from build123d import *

# Parameters (mm, degrees)
SKETCH_1_W          = 18
SKETCH_1_H          = 18
EXTRUDE_1_DEPTH     = 25
SKETCH_2_R          = 6.55
CUT_EXTRUDE_1_DEPTH = 4.5
CUT_EXTRUDE_2_DEPTH = 11.7
CUT_EXTRUDE_3_DEPTH = 16
SKETCH_6_W          = 18
SKETCH_6_H          = 18
SKETCH_6_W_2        = 17
SKETCH_6_H_2        = 17
CUT_EXTRUDE_5_DEPTH = 26


with BuildPart() as part:
    # 草图1 → 凸台-拉伸1 (new body)
    with BuildSketch(Plane(origin=(0, 0, 0), x_dir=(0, 0, -1), z_dir=(1, 0, 0))):
        with Locations((9, 9)):
            Rectangle(SKETCH_1_W, SKETCH_1_H)
    extrude(amount=EXTRUDE_1_DEPTH)

    # 草图2 → 切除-拉伸1 (cut)
    with BuildSketch(Plane.XY):
        with Locations((10, 9)):
            Circle(SKETCH_2_R)
    extrude(amount=-CUT_EXTRUDE_1_DEPTH, mode=Mode.SUBTRACT)

    # 草图3 → 切除-拉伸2 (cut)
    with BuildSketch(Plane.XY.offset(-4.5)):
        Polygon((10, 13.618802154), (6, 11.309401077), (6, 6.690598923), (10, 4.381197846), (14, 6.690598923), (14, 11.309401077), align=None)
    extrude(amount=-CUT_EXTRUDE_2_DEPTH, mode=Mode.SUBTRACT)

    # 草图4 → 切除-拉伸3 (cut)
    with BuildSketch(Plane.XY):
        Polygon((19, 17.886751346), (16.5, 16.443375673), (16.5, 13.556624327), (19, 12.113248654), (21.5, 13.556624327), (21.5, 16.443375673), align=None)
    extrude(amount=-CUT_EXTRUDE_3_DEPTH, mode=Mode.SUBTRACT)

    # 草图6 → 切除-拉伸5 (cut, through all)
    with BuildSketch(Plane.ZY):
        with Locations((-9, 9)):
            Rectangle(SKETCH_6_W, SKETCH_6_H)
        with Locations((-9, 9)):
            Rectangle(SKETCH_6_W_2, SKETCH_6_H_2, mode=Mode.SUBTRACT)
    extrude(amount=-CUT_EXTRUDE_5_DEPTH, mode=Mode.SUBTRACT)


solid = part.part
Read the model definition and answer for the solid it produces. Units are mm, in the model's axes. A direction names the side the tool comes from. Round coordinates to 2 decimals unless told otherwise and drop trailing zeros. Write each loop counter-clockwise with the first axis right and the second up, starting at its lowest first coordinate (ties: lowest second). Pieces come first, ordered by that corner, then holes. Notation, with made-up numbers: (0, -17) - (10, -17) arc R23 ccw to (10, -7) - close; hole circle Ø7 at (23, 21.25). An arc over 180 degrees is marked (long way). Use a Markdown table: item, result.
(1) Straight lines are drawn through the part: line 1 along X through (y, z) = (11, -7.5); line 2 along X through (y, z) = (12.75, -13.5); line 3 along Y through (x, z) = (10, -3.05). For each, find the intervals that lie inside material, in ascending order. Write a range as [from, to].
Reported:
| item | result |
|---|---|
| line 1 | [0, 6], [14, 25] |
| line 2 | [0, 8.5], [11.5, 17.9], [20.1, 25] |
| line 3 | [0.5, 2.45], [15.55, 17.5] |
(2) The part is cut by section C-C (x = 20). Write down the section's boundary in (y, z).
Reported:
| item | result |
|---|---|
| outline | (0.5, -17.5) - (17.5, -17.5) - (17.5, -0.5) - (17.31, -0.5) - (17.31, -16) - (12.69, -16) - (12.69, -0.5) - (0.5, -0.5) - close |
(3) The part is cut by section A-A (z = -2.75). Write down the section's boundary in (x, y).
Reported:
| item | result |
|---|---|
| outline | (0, 0.5) - (25, 0.5) - (25, 17.5) - (19.67, 17.5) - (21.5, 16.44) - (21.5, 13.56) - (19, 12.11) - (16.5, 13.56) - (16.5, 16.44) - (18.33, 17.5) - (0, 17.5) - close; hole circle Ø13.1 at (10, 9) |
(4) The part is cut by section D-D (z = -10.5). Write down the section's boundary in (x, y).
Reported:
| item | result |
|---|---|
| outline | (0, 0.5) - (25, 0.5) - (25, 17.5) - (19.67, 17.5) - (21.5, 16.44) - (21.5, 13.56) - (19, 12.11) - (16.5, 13.56) - (16.5, 16.44) - (18.33, 17.5) - (0, 17.5) - close; hole (6, 6.69) - (10, 4.38) - (14, 6.69) - (14, 11.31) - (10, 13.62) - (6, 11.31) - close |
(5) Each of these flat-tipped pins is pushed along its axis until it touches: pin 1 Ø4 at (x, y) = (10, 11) entering from +Z; pin 2 Ø4 at (x, y) = (11.5, 6) entering from +Z. Where does it stop, or does it pass through?
Reported:
| item | result |
|---|---|
| pin 1 | z = -16.2 |
| pin 2 | z = -4.5 |
(6) Which of the six approach directions +Z, -Z, +X, -X, +Y, -Y give full straight-line access (tool end or side, diameter ignored) to faces 5 (the flat face through (12, 17.5, -9)), 6 (the flat face through (20.598, 16.964, -8.142))?
Reported:
| item | result |
|---|---|
| face 5 | +Z, -Z, +X, -X, +Y |
| face 6 | +Z |
(7) The mould has two halves that part along Y. Classify faces 1 (the flat face through (18, 9, -0.5)), 2 (the flat face through (8.03, 12.48, -10.27)), 3 (the flat face through (12.028, 12.448, -10.268)), 4 (the flat face through (12, 0.5, -9)): released by +Y, released by -Y, zero draft, split by the parting line, or undercut.
Reported:
| item | result |
|---|---|
| face 1 | zero draft |
| face 2 | undercut |
| face 3 | undercut |
| face 4 | released by -Y |
(8) The part is cut by section B-B (y = 6). Write down the section's boundary in (x, z), then the cut area to 3 significant figures.
Reported:
| item | result |
|---|---|
| outline | (0, -17.5) - (25, -17.5) - (25, -0.5) - (15.82, -0.5) - (15.82, -4.5) - (12.8, -4.5) - (12.8, -16.2) - (7.2, -16.2) - (7.2, -4.5) - (4.18, -4.5) - (4.18, -0.5) - (0, -0.5) - close |
| area | 313 mm2 |
